The model under review builds one solid part; all positions refer to its coordinate system, in mm. A direction names the side the tool comes from. Round coordinates to 2 decimals unless told otherwise and drop trailing zeros. Write each loop counter-clockwise with the first axis right and the second up, starting at its lowest first coordinate (ties: lowest second). Pieces come first, ordered by that corner, then holes. Notation, with made-up numbers: M -38.75,26 L -5.75,26 A26 ccw -5.75,46 Z; hole C 18,41.25 d1. An arc over 180 degrees is marked long. Write item = value, one per line. Start each with the question number.
Item 1: Take a section at D-D, the plane x = 0. Give the boundary of the cut face in (y, z), plus the area to 3 significant figures.
Item 2: Tool access review of faces 1 (the flat face through (14, -8.1, 5.5)), 2 (the flat face through (-14, -7.9, 0.5)), 3 (the flat face through (14, -8.1, 0.5)): name each direction out of +Z, -Z, +X, -X, +Y, -Y from which nothing blocks a thin tool from reaching the whole face with its end or side.
Item 3: The part is to be moulded in two halves that separate along X. For faces 4 (the flat face through (-22, -17.5, 0.5)), 5 (the flat face through (12.5, -9, 3)), 6 (the flat face through (17, -19, 5)), say which applies: +X half, -X half, draft (parallel to the pull), parting line (faces both ways), or undercut.
Item 4: To check wall thickness, follow line 1 along X through (y, z) = (-1.5, 2.25); line 2 along Z through (x, y) = (-17.5, -17.85); line 3 along X through (y, z) = (-12, 5.75). State the ranges of each line that lie inside material, in increasing order.
Item 5: For pin 1 Ø2 at (y, z) = (-14.5, 3) entering from +X; pin 2 Ø1.8 at (x, z) = (-16.5, 2.5) entering from +Y; pin 3 Ø2 at (x, z) = (5.5, 4) entering from -Y, all flat-tipped, find the tip position at first contact; note any pin that passes through.
Item 6: Take a section at B-B, the plane y = -9. Give the boundary of the cut face in (x, z).
Item 7: Take a section at A-A, the plane x = -17.5. Give the boundary of the cut face in (y, z).
Item 8: Take a section at C-C, the plane z = 3. Give the boundary of the cut face in (x, y), plus the area to 3 significant figures.
from build123d import *

# Parameters (mm, degrees)
BOSS_EXTRUDE1_DEPTH = 6
SKETCH2_R           = 1.75
CUT_EXTRUDE1_DEPTH  = 41.798284278
CHAMFER1_SIZE       = 1


with BuildPart() as part:
    # Sketch1 → Boss-Extrude1 (new body)
    with BuildSketch(Plane.XY):
        with BuildLine():
            Line((-14.5, 0), (-14.5, -16))
            Line((-14.5, -16), (-22.5, -16))
            Line((-22.5, -16), (-22.5, -19))
            Line((-22.5, -19), (-12.5, -19))
            Line((-12.5, -19), (-12.5, 0))
            ThreePointArc((-12.5, 0), (0, 12.5), (12.5, 0))
            Line((12.5, 0), (12.5, -19))
            Line((12.5, -19), (22.5, -19))
            Line((22.5, -19), (22.5, -16))
            Line((22.5, -16), (14.5, -16))
            Line((14.5, -16), (14.5, 0))
            ThreePointArc((14.5, 0), (0, 14.5), (-14.5, 0))
        make_face()
    extrude(amount=BOSS_EXTRUDE1_DEPTH)

    # Sketch2 → Cut-Extrude1 (cut, through all)
    with BuildSketch(Plane.XZ.offset(19)):
        with Locations((-17.5, 3)):
            Circle(SKETCH2_R)
        with Locations((17.5, 3)):
            Circle(SKETCH2_R)
    extrude(amount=-CUT_EXTRUDE1_DEPTH, mode=Mode.SUBTRACT)

    # Chamfer1
    chamfer1_edges = [part.edges().sort_by_distance(p)[0] for p in [
        (14.5, -8, 0),
        (22.5, -17.5, 0),
        (-22.5, -17.5, 0),
        (-14.5, -8, 0),
        (0, 14.5, 0),
        (-22.5, -17.5, 6),
        (22.5, -17.5, 6),
        (14.5, -8, 6),
        (0, 14.5, 6),
        (-14.5, -8, 6),
    ]]
    chamfer(chamfer1_edges, length=CHAMFER1_SIZE)


solid = part.part
Response values:
q1.outline = M 12.5,0 L 13.5,0 L 14.5,1 L 14.5,5 L 13.5,6 L 12.5,6 Z
q1.area = 11.0 mm2
q2.face_1 = +Z, +X, +Y
q2.face_2 = -Z, -X, +Y
q2.face_3 = -Z, +X, +Y
q3.face_4 = -X half
q3.face_5 = undercut
q3.face_6 = draft
q4.line_1 = -14.5 to -12.5, 12.5 to 14.5
q4.line_2 = 0 to 1.25, 4.75 to 6
q4.line_3 = -13.75 to -12.5, 12.5 to 13.75
q5.pin_1 = 14.5
q5.pin_2 = -16
q5.pin_3 = 10.68
q6.outline = M -14.5,1 L -13.5,0 L -12.5,0 L -12.5,6 L -13.5,6 L -14.5,5 Z; M 12.5,0 L 13.5,0 L 14.5,1 L 14.5,5 L 13.5,6 L 12.5,6 Z
q7.outline = M -19,0 L -16,0 L -16,1.25 L -19,1.25 Z; M -19,4.75 L -16,4.75 L -16,6 L -19,6 Z
q8.outline = M -22.5,-19 L -19.25,-19 L -19.25,-16 L -22.5,-16 Z; M -15.75,-19 L -12.5,-19 L -12.5,0 A12.5 cw 12.5,0 L 12.5,-19 L 15.75,-19 L 15.75,-16 L 14.5,-16 L 14.5,0 A14.5 ccw -14.5,0 L -14.5,-16 L -15.75,-16 Z; M 19.25,-19 L 22.5,-19 L 22.5,-16 L 19.25,-16 Z
q8.area = 188 mm2
